Verification items for the finished model (mm, model axes). Face numbers are marked on the shaded views. A direction names the side the tool comes from. Round coordinates to 2 decimals unless told otherwise and drop trailing zeros. Loops run counter-clockwise (first coordinate to the right, second up) from the corner with the lowest first, then second, coordinate; pieces in that order, holes last. Notation, with made-up numbers: M 83,33 L 125,33 A8 ccw 125,41 Z; hole C -6.75,-16.75 d3. An arc over 180 degrees is marked long. Answer as CSV lines item,"result".
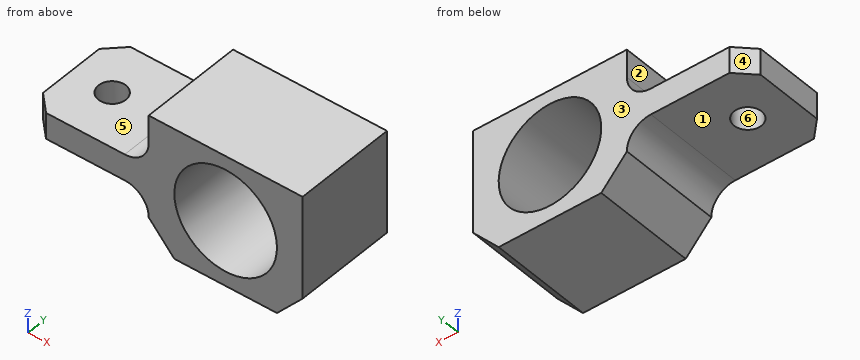
```python
from build123d import *

# Parameters (mm, degrees)
EXTRUDE_1_DEPTH     = 30
SKETCH_2_R          = 15
CUT_EXTRUDE_2_DEPTH = 43.140141425
SKETCH_3_W          = 7.64
SKETCH_3_H          = 30
EXTRUDE_3_DEPTH     = 35
CHAMFER_1_SIZE      = 5
SKETCH_5_R          = 4
CUT_EXTRUDE_4_DEPTH = 69.827691917
FILLET_2_R          = 7
FILLET_3_R          = 7


with BuildPart() as part:
    # Эскиз1 → Вытянуть1 (new body)
    with BuildSketch(Plane(origin=(0, 0, 0), x_dir=(1, 0, 0), z_dir=(0, 1, 0))):
        Polygon((22.5, -19.019063342), (-22.5, -19.019063342), (-22.5, 10.980936658), (-15, 19.22346273), (15, 19.22346273), (22.5, 10.980936658), align=None)
    extrude(amount=EXTRUDE_1_DEPTH)

    # Эскиз2 → Вытянуть2 (cut, through all)
    with BuildSketch(Plane(origin=(0, 30, 0), x_dir=(1, 0, 0), z_dir=(0, 1, 0))):
        with Locations(Location((0, 0, 0), (0, 0, 270))):
            Circle(SKETCH_2_R)
    extrude(amount=-CUT_EXTRUDE_2_DEPTH, mode=Mode.SUBTRACT)

    # Эскиз3 → Вытянуть3 (add)
    with BuildSketch(Plane.ZY.offset(22.5)):
        with Locations((0, 15)):
            Rectangle(SKETCH_3_W, SKETCH_3_H)
    extrude(amount=EXTRUDE_3_DEPTH)

    # Фаска1
    chamfer_1_edges = [part.edges().sort_by_distance(p)[0] for p in [
        (-57.5, 0, 0),
        (-57.5, 30, 0),
    ]]
    chamfer(chamfer_1_edges, length=CHAMFER_1_SIZE)

    # Эскиз5 → Вытянуть4 (cut, through all)
    with BuildSketch(Plane.XY.offset(3.82)):
        with Locations((-45.5, 15)):
            Circle(SKETCH_5_R)
    extrude(amount=-CUT_EXTRUDE_4_DEPTH, mode=Mode.SUBTRACT)

    # Скругление2
    fillet_2_edges = [part.edges().sort_by_distance(p)[0] for p in [
        (-22.5, 15, -3.82),
    ]]
    fillet(fillet_2_edges, radius=FILLET_2_R)

    # Скругление3
    fillet_3_edges = [part.edges().sort_by_distance(p)[0] for p in [
        (-22.5, 15, 3.82),
    ]]
    fillet(fillet_3_edges, radius=FILLET_3_R)


solid = part.part
```
1) Material ranges on probe 1 along Y at (x, z) = (-45.5, -1.75); probe 2 along X at (y, z) = (8, 0); probe 3 along X at (y, z) = (18, 11), recorded low to high.
Here are the results:
probe 1,"y = 0 to 11, 19 to 30"
probe 2,"x = -57.5 to -15, 15 to 22.5"
probe 3,"x = -22.5 to -10.2, 10.2 to 22.5"
2) Set-up check for the marked faces 1, 2 and 3: record each of +Z, -Z, +X, -X, +Y, -Y from which the full face is reachable in a straight line by a thin tool's end or side.
Here are the results:
face 1,"-Z, -X, +Y, -Y"
face 2,"+Z, -X, +Y, -Y"
face 3,"+Z, -Z, +X, -X, +Y"
3) Draft check along Y on the marked faces 4, 5 and 6. Enter one of: +Y half, -Y half, draft (parallel to the pull), parting line (faces both ways), or undercut.
Here are the results:
face 4,"+Y half"
face 5,"draft"
face 6,"undercut"
4) Section check D-D (y = 23.5). Record the cut outline in (x, z), plus the area to 3 significant figures.
Here are the results:
outline,"M -57.5,-3.82 L -29.5,-3.82 A7 cw -22.5,-10.82 L -22.5,-10.98 L -15,-19.22 L 15,-19.22 L 22.5,-10.98 L 22.5,19.02 L -22.5,19.02 L -22.5,10.82 A7 cw -29.5,3.82 L -57.5,3.82 Z; hole C 0,0 d30"
area,"1,240 mm^2"
5) Go/stop test with flat-tipped pins: pin 1 (8.5 mm diameter, centred on x = -42, y = 7.5, fed in from +Z); pin 2 (4 mm diameter, centred on x = -48, y = 16.5, fed in from -Z); pin 3 (2.5 mm diameter, centred on y = 18, z = 15, fed in from -X). Record where each tip stops, or that it passes through.
Here are the results:
pin 1,"stops at z = 3.82"
pin 2,"stops at z = -3.82"
pin 3,"stops at x = -22.5"
6) Section check B-B (z = 0). Record the cut outline in (x, y).
Here are the results:
outline,"M -57.5,5 L -52.5,0 L -15,0 L -15,30 L -52.5,30 L -57.5,25 Z; M 15,0 L 22.5,0 L 22.5,30 L 15,30 Z; hole C -45.5,15 d8"
7) Section check A-A (y = 15). Record the cut outline in (x, z).
Here are the results:
outline,"M -57.5,-3.82 L -49.5,-3.82 L -49.5,3.82 L -57.5,3.82 Z; M -41.5,-3.82 L -29.5,-3.82 A7 cw -22.5,-10.82 L -22.5,-10.98 L -15,-19.22 L 15,-19.22 L 22.5,-10.98 L 22.5,19.02 L -22.5,19.02 L -22.5,10.82 A7 cw -29.5,3.82 L -41.5,3.82 Z; hole C 0,0 d30"
8) Section check C-C (x = 0). Record the cut outline in (y, z).
Here are the results:
outline,"M 0,-19.22 L 30,-19.22 L 30,-15 L 0,-15 Z; M 0,15 L 30,15 L 30,19.02 L 0,19.02 Z"
